The listing builds one solid part. Answer for the finished solid, in the listing's coordinates (mm). A direction names the side the tool comes from. Coordinates: 2 decimals unless noted, no trailing zeros. Loops run counter-clockwise (first coordinate to the right, second up) from the corner with the lowest first, then second, coordinate; pieces in that order, holes last. Notation, with made-up numbers: (83, 38) - (120, 38) arc R18 ccw to (120, 52) - close; hole circle Ø4 at (12, -17). An arc over 180 degrees is marked (long way). Use one line per item in the form item = value. Start each with the question number.
```python
from build123d import *

# Parameters (mm, degrees)
SKETCH1_W               = 75
SKETCH1_H               = 50
BOSS_EXTRUDE1_DEPTH     = 10
BOSS_EXTRUDE2_DEPTH     = 10
FILLET1_R               = 10
SKETCH4_R               = 5
CUT_EXTRUDE1_DEPTH      = 5
FILLET1_OF_MIRROR1_R    = 10
SKETCH5_R               = 2.5625
CUT_EXTRUDE2_DEPTH      = 11
MIRROR3_COPY_1_SKETCH_R = 2.5625
MIRROR3_COPY_1_DEPTH    = 11
SKETCH6_W               = 30
SKETCH6_H               = 30
CUT_EXTRUDE3_DEPTH      = 5


with BuildPart() as part:
    # Sketch1 → Boss-Extrude1 (new body)
    with BuildSketch(Plane(origin=(0, 0, 0), x_dir=(1, 0, 0), z_dir=(0, 1, 0))):
        with Locations((37.5, 25)):
            Rectangle(SKETCH1_W, SKETCH1_H)
    extrude(amount=BOSS_EXTRUDE1_DEPTH)

    # Sketch2 → Boss-Extrude2 (add)
    with BuildSketch(Plane.XY):
        with BuildLine():
            Line((52.5, 20), (57.5, 10))
            Line((57.5, 10), (17.5, 10))
            Line((17.5, 10), (22.5, 20))
            ThreePointArc((22.5, 20), (37.5, 35), (52.5, 20))
        make_face()
    boss_extrude2 = extrude(amount=-BOSS_EXTRUDE2_DEPTH)

    # Fillet1
    fillet1_edges = [part.edges().sort_by_distance(p)[0] for p in [
        (22.5, 20, -5),
        (52.5, 20, -5),
        (57.5, 10, -5),
        (17.5, 10, -5),
    ]]
    fillet(fillet1_edges, radius=FILLET1_R)

    # Sketch4 → Cut-Extrude1 (cut)
    with BuildSketch(Plane(origin=(0, 0, -10), x_dir=(-1, 0, 0), z_dir=(0, 0, -1))):
        with Locations((-37.5, 20)):
            Circle(SKETCH4_R)
    cut_extrude1 = extrude(amount=-CUT_EXTRUDE1_DEPTH, mode=Mode.SUBTRACT)

    # Mirror1: Boss-Extrude2, Cut-Extrude1 across plane
    add(boss_extrude2.mirror(Plane(origin=(0, 0, -25), x_dir=(1, 0, 0), z_dir=(0, 0, -1))))
    add(cut_extrude1.mirror(Plane(origin=(0, 0, -25), x_dir=(1, 0, 0), z_dir=(0, 0, -1))), mode=Mode.SUBTRACT)

    # Fillet1 of Mirror1
    fillet1_of_mirror1_edges = [part.edges().sort_by_distance(p)[0] for p in [
        (22.5, 20, -45),
        (52.5, 20, -45),
        (57.5, 10, -45),
        (17.5, 10, -45),
    ]]
    fillet(fillet1_of_mirror1_edges, radius=FILLET1_OF_MIRROR1_R)

    # Sketch5 → Cut-Extrude2 (cut, through all)
    with BuildSketch(Plane(origin=(0, 10, 0), x_dir=(1, 0, 0), z_dir=(0, 1, 0))):
        with Locations((5, 5)):
            Circle(SKETCH5_R)
    cut_extrude2 = extrude(amount=-CUT_EXTRUDE2_DEPTH, mode=Mode.SUBTRACT)

    # Mirror2: Cut-Extrude2 across plane
    add(cut_extrude2.mirror(Plane(origin=(0, 0, -25), x_dir=(1, 0, 0), z_dir=(0, 0, -1))), mode=Mode.SUBTRACT)

    # Mirror3: Cut-Extrude2 across plane
    add(cut_extrude2.mirror(Plane(origin=(37.5, 0, 0), x_dir=(0, 0, 1), z_dir=(1, 0, 0))), mode=Mode.SUBTRACT)

    # Mirror3 copy 1 sketch → Mirror3 copy 1 (cut, through all)
    with BuildSketch(Plane(origin=(75, 10, -50), x_dir=(-1, 0, 0), z_dir=(0, 1, 0))):
        with Locations((5, 5)):
            Circle(MIRROR3_COPY_1_SKETCH_R)
    extrude(amount=-MIRROR3_COPY_1_DEPTH, mode=Mode.SUBTRACT)

    # Sketch6 → Cut-Extrude3 (cut)
    with BuildSketch(Plane(origin=(0, 10, 0), x_dir=(1, 0, 0), z_dir=(0, 1, 0))):
        with Locations((37.5, 25)):
            Rectangle(SKETCH6_W, SKETCH6_H)
    extrude(amount=-CUT_EXTRUDE3_DEPTH, mode=Mode.SUBTRACT)


solid = part.part
```
(1) A cutting plane is placed at A-A (x = 5). Determine the outline of the cut face in (y, z), then the cut area to 4 significant figures.
(2) Find the intervals of material crossed by probe 1 along X at (y, z) = (2.5, -5); probe 2 along Z at (x, y) = (5, 4); probe 3 along Z at (x, y) = (40.5, 13), in increasing order. Write a range as from..to.
(3) Each of these flat-tipped pins is pushed along its axis until it touches: pin 1 Ø6.5 at (x, z) = (5, -5) entering from +Y; pin 2 Ø8 at (x, z) = (28, -22) entering from +Y. Where does it stop, or does it pass through?
(4) A cutting plane is placed at C-C (y = 29). Determine the outline of the cut face in (x, z), then the cut area to 3 significant figures.
(5) Determine the mould class of faces 4 (the face through (72.56, 5.07, -5.11)), 5 (the face through (38, 20, -45)), 6 (the face through (0, 5, -25)), 7 (the face through (58.489, 11.453, -5.07)) for opening direction X: +X half, -X half, draft (parallel to the pull), parting line (faces both ways), or undercut.
(6) A cutting plane is placed at D-D (z = -28). Determine the outline of the cut face in (x, y), then the cut area to 3 significant figures.
(7) A cutting plane is placed at B-B (y = 2). Determine the outline of the cut face in (x, z) (1 decimal).
(8) For faces 1 (the face through (54, 17, -5)), 2 (the face through (22.5, 8, -25)), 3 (the face through (38, 20, -5)), determine the directions among +Z, -Z, +X, -X, +Y, -Y from which every point of the face is accessible in a straight line to the end or side of a thin tool.
Evaluation:
q1.outline = (0, -50) - (10, -50) - (10, -47.56) - (0, -47.56) - close; (0, -42.44) - (10, -42.44) - (10, -7.56) - (0, -7.56) - close; (0, -2.44) - (10, -2.44) - (10, 0) - (0, 0) - close
q1.area = 397.5 mm^2
q2.probe_1 = 0..2.44, 7.56..67.44, 72.56..75
q2.probe_2 = -50..-47.56, -42.44..-7.56, -2.44..0
q2.probe_3 = -50..-40, -10..0
q3.pin_1 = 10
q3.pin_2 = 5
q4.outline = (25.5, -50) - (49.5, -50) - (49.5, -40) - (25.5, -40) - close; (25.5, -10) - (49.5, -10) - (49.5, 0) - (25.5, 0) - close
q4.area = 480 mm^2
q5.face_4 = undercut
q5.face_5 = undercut
q5.face_6 = -X half
q5.face_7 = +X half
q6.outline = (0, 0) - (75, 0) - (75, 10) - (52.5, 10) - (52.5, 5) - (22.5, 5) - (22.5, 10) - (0, 10) - close
q6.area = 600 mm^2
q7.outline = (0, -50) - (75, -50) - (75, 0) - (0, 0) - close; hole circle Ø5.1 at (5, -45); hole circle Ø5.1 at (5, -5); hole circle Ø5.1 at (70, -45); hole circle Ø5.1 at (70, -5)
q8.face_1 = +Z, -Z, +X, +Y
q8.face_2 = +Y
q8.face_3 = none
